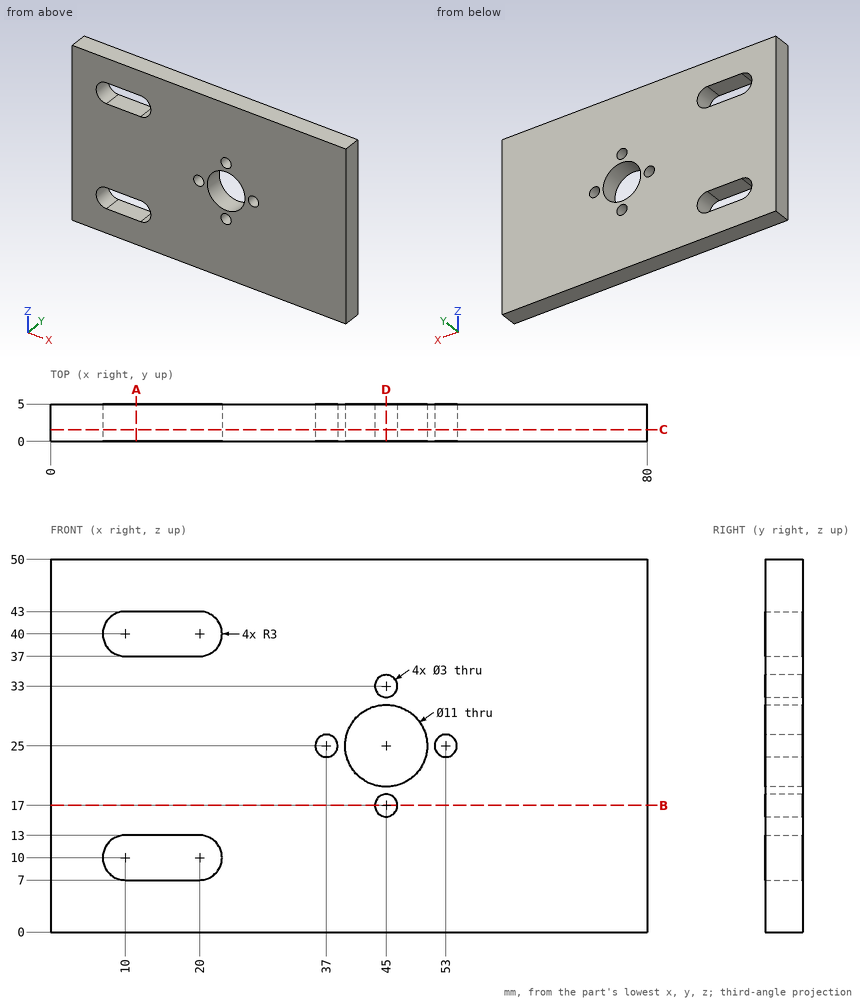
Verification items for this drawing (mm, ordinates from the low corner). Give positions to 0.01 mm unless a question says otherwise; leave off trailing zeros. Order: outer loops, then holes, each group sorted by start corner. A loop starts at its lowest first (then second) coordinate and runs counter-clockwise, first axis right, second up. Notation, with made-up numbers: M 69.25,33.5 L 120.25,33.5 A16 ccw 120.25,56.5 Z; hole C -28,61 d11. An arc over 180 degrees is marked long. Use a Markdown table: item, result.
Item 1: Section check A-A (x = 11.5). Record the cut outline in (y, z).
Answers follow:
| item | result |
|---|---|
| outline | M 0,0 L 5,0 L 5,7 L 0,7 Z; M 0,13 L 5,13 L 5,37 L 0,37 Z; M 0,43 L 5,43 L 5,50 L 0,50 Z |
Item 2: Section check B-B (z = 17). Record the cut outline in (x, y), and give its area (3 significant figures).
Answers follow:
| item | result |
|---|---|
| outline | M 0,0 L 43.5,0 L 43.5,5 L 0,5 Z; M 46.5,0 L 80,0 L 80,5 L 46.5,5 Z |
| area | 385 mm2 |
Item 3: Section check C-C (y = 1.55). Record the cut outline in (x, z).
Answers follow:
| item | result |
|---|---|
| outline | M 0,0 L 80,0 L 80,50 L 0,50 Z; hole M 10,7 L 20,7 A3 ccw 20,13 L 10,13 A3 ccw Z; hole M 10,37 L 20,37 A3 ccw 20,43 L 10,43 A3 ccw Z; hole C 37,25 d3; hole C 45,25 d11; hole C 45,17 d3; hole C 45,33 d3; hole C 53,25 d3 |
Item 4: Section check D-D (x = 45). Record the cut outline in (y, z).
Answers follow:
| item | result |
|---|---|
| outline | M 0,0 L 5,0 L 5,15.5 L 0,15.5 Z; M 0,18.5 L 5,18.5 L 5,19.5 L 0,19.5 Z; M 0,30.5 L 5,30.5 L 5,31.5 L 0,31.5 Z; M 0,34.5 L 5,34.5 L 5,50 L 0,50 Z |
Item 5: Material ranges on line 1 along Z through (x, y) = (15.5, 0.9); line 2 along X through (y, z) = (1.15, 25); line 3 along Z through (x, y) = (53, 2.75), recorded low to high.
Answers follow:
| item | result |
|---|---|
| line 1 | z = 0 to 7, 13 to 37, 43 to 50 |
| line 2 | x = 0 to 35.5, 38.5 to 39.5, 50.5 to 51.5, 54.5 to 80 |
| line 3 | z = 0 to 23.5, 26.5 to 50 |
